Autodesk Fusion 360 part; units mm, degrees
sketch "Sketch1" plane through (0, 0, 0) normal (0, 0, 1) x (1, 0, 0)
  line L0 (0, 0) -> (64, 0)
  line L1 (64, 0) -> (64, 37)
  line L2 (64, 37) -> (0, 37)
  line L3 (0, 37) -> (0, 0)
  dimension "d1" = 64
  dimension "d2" = 37
extrude "Extrude1" add sketch "Sketch1" along normal blind 16
fillet "Fillet1" radius 3 4 edges at (32, 0, 16) (32, 37, 16) (32, 0, 0) (32, 37, 0)
fillet "Fillet2" radius 0.5 16 edges at (64, 36.1213, 0.8787) (64, 37, 8) (64, 36.1213, 15.1213) (64, 18.5, 16) (64, 0.8787, 15.1213) (64, 0, 8) (64, 0.8787, 0.8787) (64, 18.5, 0) (0, 0.8787, 0.8787) (0, 0, 8) (0, 0.8787, 15.1213) (0, 18.5, 16) (0, 36.1213, 15.1213) (0, 37, 8) (0, 36.1213, 0.8787) (0, 18.5, 0)
sketch "Sketch2" plane through (0, 0, 16) normal (0, 0, 1) x (-1, 0, 0)
  line L0 (-0.5, -34) -> (-0.5, -3)
  line L1 (-0.5, -3) -> (-63.5, -3)
  line L2 (-63.5, -3) -> (-63.5, -34)
  line L3 (-63.5, -34) -> (-0.5, -34)
  line L4 (-5, -24) -> (-8, -24)
  line L5 (-8, -24) -> (-8, -30)
  line L6 (-8, -30) -> (-5, -30)
  line L7 (-5, -30) -> (-5, -24)
  dimension "d7" = 3
  dimension "d8" = 6
extrude "Extrude2" cut sketch "Sketch2" against normal blind 0.5 contours L4 L5 L6 L7
sketch "Sketch3" plane through (0, 0, 15.5) normal (0, 0, 1) x (-1, 0, 0)
  line L0 (-5, -30) -> (-5, -24)
  line L1 (-5, -24) -> (-8, -24)
  line L2 (-8, -24) -> (-8, -30)
  line L3 (-8, -30) -> (-5, -30)
  line L4 (-5, -27) -> (-8, -27)
  line L5 (-5.1, -27.1) -> (-7.9, -27.1)
  line L6 (-7.9, -27.1) -> (-7.9, -29.9)
  line L7 (-7.9, -29.9) -> (-5.1, -29.9)
  line L8 (-5.1, -29.9) -> (-5.1, -27.1)
extrude "Extrude3" add sketch "Sketch3" along normal blind 2 contours L5 L6 L7 L8
For this review, take the finished solid that the model builds, in its own axes (mm). A direction names the side the tool comes from. Coordinates: 2 decimals unless noted, no trailing zeros. Loops run counter-clockwise (first coordinate to the right, second up) from the corner with the lowest first, then second, coordinate; pieces in that order, holes last. Notation, with made-up numbers: (-8.75, 69.5) -> (29.25, 69.5) arc R14 ccw to (29.25, 92.5) -> close; hole circle Ø11 at (53, -33). An arc over 180 degrees is marked (long way). Write each question's results on one line, items separated by ' | '.
Q1. Machinability: for faces 1 (the flat face through (5.1, 28.5, 16.5)), 2 (the flat face through (7, 28, 17.5)), which of the approach directions +Z, -Z, +X, -X, +Y, -Y give a long, thin tool a straight path to every point of the face, cutting with its end or side? Answer none if there is none.
Taken from the geometry:
face 1: +Z | face 2: +Z, +X, -X, +Y, -Y
Q2. To check wall thickness, follow line 1 along Z through (x, y) = (47.5, 10); line 2 along Y through (x, z) = (6, 16.75); line 3 along Y through (x, z) = (23.5, 2.75). State the ranges of each line that lie inside material, in increasing order. Write a range as [from, to].
Taken from the geometry:
line 1: [0, 16] | line 2: [27.1, 29.9] | line 3: [0.01, 36.99]
Q3. Add section C-C, the plane y = 20. State the section outline as (x, z) points.
Taken from the geometry:
outline: (0, 0.5) arc R0.5 ccw to (0.5, 0) -> (63.5, 0) arc R0.5 ccw to (64, 0.5) -> (64, 15.5) arc R0.5 ccw to (63.5, 16) -> (0.5, 16) arc R0.5 ccw to (0, 15.5) -> close
Q4. Add section B-B, the plane x = 42. State the section outline as (y, z) points, then the cut area to 3 significant figures.
Taken from the geometry:
outline: (0, 3) arc R3 ccw to (3, 0) -> (34, 0) arc R3 ccw to (37, 3) -> (37, 13) arc R3 ccw to (34, 16) -> (3, 16) arc R3 ccw to (0, 13) -> close | area: 584 mm²
Q5. Mouldability with a two-part tool opening along Y and no side actions: class faces 3 (the cylindrical face through (31.56, 36.14, 0.9)), 4 (the flat face through (32, 19, 16)), 5 (the flat face through (7, 26, 15.5)) as +Y half, -Y half, draft (parallel to the pull), parting line (faces both ways), or undercut.
Taken from the geometry:
face 3: +Y half | face 4: draft | face 5: undercut
Q6. For pin 1 Ø1.5 at (x, y) = (6.5, 26) entering from +Z; pin 2 Ø0.6 at (y, z) = (28.5, 16.5) entering from +X; pin 3 Ø0.6 at (y, z) = (27.5, 16) entering from -X, all flat-tipped, find the tip position at first contact; note any pin that passes through.
Taken from the geometry:
pin 1: z = 15.5 | pin 2: x = 7.9 | pin 3: x = 0.04
Q7. Add section A-A, the plane y = 26. State the section outline as (x, z) points, then the cut area to 3 significant figures.
Taken from the geometry:
outline: (0, 0.5) arc R0.5 ccw to (0.5, 0) -> (63.5, 0) arc R0.5 ccw to (64, 0.5) -> (64, 15.5) arc R0.5 ccw to (63.5, 16) -> (8, 16) -> (8, 15.5) -> (5, 15.5) -> (5, 16) -> (0.5, 16) arc R0.5 ccw to (0, 15.5) -> close | area: 1,020 mm²
